Read the model definition and answer for the solid it produces. Units are mm, in the model's axes. A direction names the side the tool comes from. Coordinates: 2 decimals unless noted, no trailing zeros. Loops run counter-clockwise (first coordinate to the right, second up) from the corner with the lowest first, then second, coordinate; pieces in that order, holes last. Notation, with made-up numbers: (40.5, -19) -> (67.5, -19) arc R32 ccw to (67.5, 9) -> close; hole circle Ø4 at (31, 47). An arc over 180 degrees is marked (long way). Answer as a JSON object with one key per item and string values. Group by question number.
Q1. The part is cut by section A-A on x = 24. Write down the section's boundary in (y, z), and give its area (3 significant figures).
Q2. Each of these flat-tipped pins is pushed along its axis until it touches: P1, Ø5, axis at x = 24, z = -5, coming from the +Y side; P2, Ø4.5, axis at x = -24, z = -5, coming from the -Y side; P3, Ø2, axis at x = -19, z = 8.5, coming from the +Y side; P4, Ø3.5, axis at x = 24, z = 5, coming from the +Y side. Where does it stop, or does it pass through?
Q3. The part is cut by section D-D on z = 1.5. Write down the section's boundary in (x, y), and give its area (3 significant figures).
Q4. Determine the mould class of faces 1 (the cylindrical face through (-22.017, 30.603, -5.26)), 2 (the flat face through (23, 31.096, 0)), 3 (the cylindrical face through (-18.6, 38.51, -8.57)) for opening direction X: released by +X, released by -X, zero draft, split by the parting line, or undercut.
Q5. Straight lines are drawn through the part: line 1 along X through (y, z) = (30.55, 5); line 2 along Y through (x, z) = (-4, 5.5); line 3 along X through (y, z) = (20.5, -4.25). For each, find the intervals that lie inside material, in ascending order. Write a range as [from, to].
Q6. The part is cut by section B-B on y = 22. Write down the section's boundary in (x, z).
Q7. For faces 4 (the flat face through (-20, 34, 0)), 5 (the flat face through (20, 34, 0)), 6 (the flat face through (20, 15, 0)), determine the directions among +Z, -Z, +X, -X, +Y, -Y from which every point of the face is accessible in a straight line to the end or side of a thin tool.
Q8. The part is cut by section C-C on x = -10. Write down the section's boundary in (y, z).
from build123d import *

# Parameters (mm, degrees)
SKETCH_1_W          = 40
SKETCH_1_H          = 10
EXTRUDE_2_DEPTH     = 39
SKETCH_4_W          = 10
SKETCH_4_H          = 1
EXTRUDE_8_DEPTH     = 8
SKETCH_12_W         = 10
SKETCH_12_H         = 1
EXTRUDE_9_DEPTH     = 8
SKETCH_14_W         = 40
SKETCH_14_H         = 20
EXTRUDE_10_DEPTH    = 39
SKETCH_15_W         = 20
SKETCH_15_H         = 1
EXTRUDE_12_DEPTH    = 8
SKETCH_16_W         = 20
SKETCH_16_H         = 1
EXTRUDE_13_DEPTH    = 8
SKETCH_17_R         = 6
EXTRUDE_15_DEPTH    = 0.75
SKETCH_19_R         = 4.98600358
EXTRUDE_16_DEPTH    = 0.25
SKETCH_20_R         = 3
EXTRUDE_17_DEPTH    = 5
SKETCH_22_R         = 2
CUT_EXTRUDE_1_DEPTH = 5
SKETCH_23_R         = 2
CUT_EXTRUDE_3_DEPTH = 5
FILLET_12_R         = 1
FILLET_13_R         = 1
SKETCH_27_R         = 2
CUT_EXTRUDE_4_DEPTH = 1
FILLET_14_R         = 1
FILLET_START        = -9
FILLET_15_DEPTH     = 18
FILLET_START_2      = -19.678632008
FILLET_15_2_DEPTH   = 39.357264016
FILLET_16_R         = 1


with BuildPart() as part:
    # 草图1 → 凸台-拉伸2 (new body)
    with BuildSketch(Plane(origin=(0, 0, 0), x_dir=(1, 0, 0), z_dir=(0, 1, 0))):
        Rectangle(SKETCH_1_W, SKETCH_1_H)
    extrude(amount=EXTRUDE_2_DEPTH)

    # 草图4 → 凸台-拉伸8 (add)
    with BuildSketch(Plane.ZY.offset(20)):
        with Locations((0, 30.596439846)):
            Rectangle(SKETCH_4_W, SKETCH_4_H)
    extrude(amount=EXTRUDE_8_DEPTH)

    # 草图12 → 凸台-拉伸9 (add)
    with BuildSketch(Plane(origin=(20, 0, 0), x_dir=(0, 0, -1), z_dir=(1, 0, 0))):
        with Locations((0, 30.596439846)):
            Rectangle(SKETCH_12_W, SKETCH_12_H)
    extrude(amount=EXTRUDE_9_DEPTH)

    # 草图14 → 凸台-拉伸10 (add)
    with BuildSketch(Plane.XZ):
        Rectangle(SKETCH_14_W, SKETCH_14_H)
    extrude(amount=-EXTRUDE_10_DEPTH)

    # 草图15 → 凸台-拉伸12 (add)
    with BuildSketch(Plane.ZY.offset(20)):
        with Locations((0, 30.596439846)):
            Rectangle(SKETCH_15_W, SKETCH_15_H)
    extrude(amount=EXTRUDE_12_DEPTH)

    # 草图16 → 凸台-拉伸13 (add)
    with BuildSketch(Plane(origin=(20, 0, 0), x_dir=(0, 0, -1), z_dir=(1, 0, 0))):
        with Locations((0, 30.596439846)):
            Rectangle(SKETCH_16_W, SKETCH_16_H)
    extrude(amount=EXTRUDE_13_DEPTH)

    # 草图17 → 凸台-拉伸15 (add)
    with BuildSketch(Plane(origin=(0, 39, 0), x_dir=(1, 0, 0), z_dir=(0, 1, 0))):
        with Locations(Location((-10, 0, 0), (0, 0, 90))):
            Circle(SKETCH_17_R)
    extrude(amount=EXTRUDE_15_DEPTH)

    # 草图19 → 凸台-拉伸16 (add)
    with BuildSketch(Plane(origin=(0, 39.75, 0), x_dir=(1, 0, 0), z_dir=(0, 1, 0))):
        with Locations(Location((-10, 0, 0), (0, 0, 270))):
            Circle(SKETCH_19_R)
    extrude(amount=EXTRUDE_16_DEPTH)

    # 草图20 → 凸台-拉伸17 (add)
    with BuildSketch(Plane(origin=(0, 40, 0), x_dir=(1, 0, 0), z_dir=(0, 1, 0))):
        with Locations(Location((-10, 0, 0), (0, 0, 270))):
            Circle(SKETCH_20_R)
    extrude(amount=EXTRUDE_17_DEPTH)

    # 草图22 → 切除-拉伸1 (cut)
    with BuildSketch(Plane(origin=(0, 31.096439846, 0), x_dir=(1, 0, 0), z_dir=(0, 1, 0))):
        with Locations(Location((-24, 5, 0), (0, 0, 270))):
            Circle(SKETCH_22_R)
        with Locations(Location((-24, -5, 0), (0, 0, 270))):
            Circle(SKETCH_22_R)
    extrude(amount=-CUT_EXTRUDE_1_DEPTH, mode=Mode.SUBTRACT)

    # 草图23 → 切除-拉伸3 (cut)
    with BuildSketch(Plane(origin=(0, 31.096439846, 0), x_dir=(1, 0, 0), z_dir=(0, 1, 0))):
        with Locations(Location((24, 5, 0), (0, 0, 270))):
            Circle(SKETCH_23_R)
        with Locations(Location((24, -5, 0), (0, 0, 270))):
            Circle(SKETCH_23_R)
    extrude(amount=-CUT_EXTRUDE_3_DEPTH, mode=Mode.SUBTRACT)

    # 圆角12
    fillet_12_edges = [part.edges().sort_by_distance(p)[0] for p in [
        (0, 0, -10),
        (0, 0, 10),
        (-20, 0, 0),
        (20, 0, 0),
    ]]
    fillet(fillet_12_edges, radius=FILLET_12_R)

    # 圆角13
    # the kernel refuses this fillet: 1 mm, written as the material it takes off along each edge
    with BuildSketch(Plane(origin=(19, 1, -9), x_dir=(1, 0, 0), z_dir=(0, 0, -1))) as fillet_13_piece_1_section:
        Polygon((0, 0), (FILLET_13_R * 1.02, 0), (FILLET_13_R * 1.02, FILLET_13_R * 1.02), (0, FILLET_13_R * 1.02), align=None)
    fillet_13_piece_1 = extrude(amount=FILLET_13_R * 1.02, mode=Mode.PRIVATE)
    fillet_13_piece_1 = fillet_13_piece_1 - Plane(origin=(19, 1, -9), x_dir=(-0.7071067811865475, 0.7071067811865475, 0), z_dir=(0, 0, -1)) * Sphere(FILLET_13_R, mode=Mode.PRIVATE)
    add(fillet_13_piece_1, mode=Mode.SUBTRACT)
    with BuildSketch(Plane(origin=(19, 1, 9), x_dir=(0, 0, 1), z_dir=(1, 0, 0))) as fillet_13_piece_2_section:
        Polygon((0, 0), (FILLET_13_R * 1.02, 0), (FILLET_13_R * 1.02, FILLET_13_R * 1.02), (0, FILLET_13_R * 1.02), align=None)
    fillet_13_piece_2 = extrude(amount=FILLET_13_R * 1.02, mode=Mode.PRIVATE)
    fillet_13_piece_2 = fillet_13_piece_2 - Plane(origin=(19, 1, 9), x_dir=(0, 0.7071067811865475, -0.7071067811865475), z_dir=(1, 0, 0)) * Sphere(FILLET_13_R, mode=Mode.PRIVATE)
    add(fillet_13_piece_2, mode=Mode.SUBTRACT)
    with BuildSketch(Plane(origin=(-19, 1, -9), x_dir=(-1, 0, 0), z_dir=(0, 0, -1))) as fillet_13_piece_3_section:
        Polygon((0, 0), (FILLET_13_R * 1.02, 0), (FILLET_13_R * 1.02, -FILLET_13_R * 1.02), (0, -FILLET_13_R * 1.02), align=None)
    fillet_13_piece_3 = extrude(amount=FILLET_13_R * 1.02, mode=Mode.PRIVATE)
    fillet_13_piece_3 = fillet_13_piece_3 - Plane(origin=(-19, 1, -9), x_dir=(0.7071067811865475, 0.7071067811865475, 0), z_dir=(0, 0, -1)) * Sphere(FILLET_13_R, mode=Mode.PRIVATE)
    add(fillet_13_piece_3, mode=Mode.SUBTRACT)
    with BuildSketch(Plane(origin=(-19, 1, 9), x_dir=(0, 0, 1), z_dir=(-1, 0, 0))) as fillet_13_piece_4_section:
        Polygon((0, 0), (FILLET_13_R * 1.02, 0), (FILLET_13_R * 1.02, -FILLET_13_R * 1.02), (0, -FILLET_13_R * 1.02), align=None)
    fillet_13_piece_4 = extrude(amount=FILLET_13_R * 1.02, mode=Mode.PRIVATE)
    fillet_13_piece_4 = fillet_13_piece_4 - Plane(origin=(-19, 1, 9), x_dir=(0, 0.7071067811865475, -0.7071067811865475), z_dir=(-1, 0, 0)) * Sphere(FILLET_13_R, mode=Mode.PRIVATE)
    add(fillet_13_piece_4, mode=Mode.SUBTRACT)
    with BuildSketch(Plane(origin=(-20, 1, -10), x_dir=(1, 0, 0), z_dir=(0, 1, 0)), Plane(origin=(-20, 1, 10), x_dir=(0, 0, -1), z_dir=(0, 1, 0))) as fillet_13_piece_5:
        with BuildLine():
            CenterArc((FILLET_13_R, -FILLET_13_R), FILLET_13_R, 90, 90)
            Line((0, -FILLET_13_R), (0, 0))
            Line((0, 0), (FILLET_13_R, 0))
        make_face()
    extrude(amount=29.096439846, mode=Mode.SUBTRACT)
    with BuildSketch(Plane(origin=(20, 1, -10), x_dir=(-1, 0, 0), z_dir=(0, 1, 0)), Plane(origin=(20, 1, 10), x_dir=(0, 0, -1), z_dir=(0, 1, 0))) as fillet_13_piece_6:
        with BuildLine():
            CenterArc((FILLET_13_R, FILLET_13_R), FILLET_13_R, 180, 90)
            Line((0, FILLET_13_R), (0, 0))
            Line((0, 0), (FILLET_13_R, 0))
        make_face()
    extrude(amount=29.096439846, mode=Mode.SUBTRACT)

    # 草图27 → 切除-拉伸4 (cut)
    with BuildSketch(Plane(origin=(0, 39, 0), x_dir=(1, 0, 0), z_dir=(0, 1, 0))):
        with Locations((-20, 10)):
            Circle(SKETCH_27_R)
        with Locations((20, 10)):
            Circle(SKETCH_27_R)
        with Locations((20, -10)):
            Circle(SKETCH_27_R)
        with Locations((-20, -10)):
            Circle(SKETCH_27_R)
    extrude(amount=-CUT_EXTRUDE_4_DEPTH, mode=Mode.SUBTRACT)

    # 圆角14
    fillet_14_edges = [part.edges().sort_by_distance(p)[0] for p in [
        (-20, 34.548219923, -10),
        (20, 34.548219923, -10),
        (20, 34.548219923, 10),
        (-20, 34.548219923, 10),
    ]]
    fillet(fillet_14_edges, radius=FILLET_14_R)

    # 圆角15: read off the stored shape, not the designer's step
    # 圆角15 outline → 圆角15 (cut)
    with BuildSketch(Plane.XY.offset(FILLET_START)):
        with BuildLine():
            Line((20, 39), (19, 39))
            ThreePointArc((19, 39), (19.707106781, 38.707106781), (20, 38))
            Line((20, 38), (20, 39))
        make_face()
        with BuildLine():
            ThreePointArc((-20, 38), (-19.707106781, 38.707106781), (-19, 39))
            Line((-19, 39), (-20, 39))
            Line((-20, 39), (-20, 38))
        make_face()
    extrude(amount=FILLET_15_DEPTH, mode=Mode.SUBTRACT)

    # Fillet 15 2 outline → Fillet 15 2 (cut)
    with BuildSketch(Plane.YZ.offset(FILLET_START_2)):
        with BuildLine():
            Line((39, -10), (39, -9))
            ThreePointArc((39, -9), (38.707106781, -9.707106781), (38, -10))
            Line((38, -10), (39, -10))
        make_face()
        with BuildLine():
            ThreePointArc((38, 10), (38.707106781, 9.707106781), (39, 9))
            Line((39, 9), (39, 10))
            Line((39, 10), (38, 10))
        make_face()
    extrude(amount=FILLET_15_2_DEPTH, mode=Mode.SUBTRACT)

    # 圆角16
    fillet_16_edges = [part.edges().sort_by_distance(p)[0] for p in [
        (28, 30.596439846, -10),
        (28, 30.596439846, 10),
        (-28, 30.596439846, -10),
        (-28, 30.596439846, 10),
    ]]
    fillet(fillet_16_edges, radius=FILLET_16_R)


solid = part.part
Final values:
{
 "1": {"outline": "(30.1, -10) -> (31.1, -10) -> (31.1, -7) -> (30.1, -7) -> close; (30.1, -3) -> (31.1, -3) -> (31.1, 3) -> (30.1, 3) -> close; (30.1, 7) -> (31.1, 7) -> (31.1, 10) -> (30.1, 10) -> close", "area": "12.0 mm2"},
 "2": {"P1": "stops at y = 31.1", "P2": "stops at y = 30.1", "P3": "stops at y = 39", "P4": "passes through"},
 "3": {"outline": "(-28, 30.1) -> (-20, 30.1) -> (-20, 1) arc R1 ccw to (-19, 0) -> (19, 0) arc R1 ccw to (20, 1) -> (20, 30.1) -> (28, 30.1) -> (28, 31.1) -> (20, 31.1) -> (20, 38) arc R1 ccw to (19, 39) -> (-4.19, 39) -> (-4.19, 39.75) -> (-5.24, 39.75) -> (-5.24, 40) -> (-7.4, 40) -> (-7.4, 45) -> (-12.6, 45) -> (-12.6, 40) -> (-14.76, 40) -> (-14.76, 39.75) -> (-15.81, 39.75) -> (-15.81, 39) -> (-19, 39) arc R1 ccw to (-20, 38) -> (-20, 31.1) -> (-28, 31.1) -> close", "area": "1,610 mm2"},
 "4": {"face 1": "undercut", "face 2": "zero draft", "face 3": "released by -X"},
 "5": {"line 1": "x = [-28, -26], [-22, 22], [26, 28]", "line 2": "y = [0, 39]", "line 3": "x = [-20, 20]"},
 "6": {"outline": "(-20, -9) arc R1 ccw to (-19, -10) -> (19, -10) arc R1 ccw to (20, -9) -> (20, 9) arc R1 ccw to (19, 10) -> (-19, 10) arc R1 ccw to (-20, 9) -> close"},
 "7": {"face 4": "+Z, -Z, -X, +Y", "face 5": "+Z, -Z, +X, +Y", "face 6": "+Z, -Z, +X, -Y"},
 "8": {"outline": "(0, -9) arc R1 ccw to (1, -10) -> (38, -10) arc R1 ccw to (39, -9) -> (39, -6) -> (39.75, -6) -> (39.75, -4.99) -> (40, -4.99) -> (40, -3) -> (45, -3) -> (45, 3) -> (40, 3) -> (40, 4.99) -> (39.75, 4.99) -> (39.75, 6) -> (39, 6) -> (39, 9) arc R1 ccw to (38, 10) -> (1, 10) arc R1 ccw to (0, 9) -> close"}
}
